Geometry check sheet. Reference: drawing and pictorial views, mm from the part's lowest x, y, z. Round coordinates to 2 decimals unless told otherwise and drop trailing zeros. Order: outer loops, then holes, each group sorted by start corner. A loop starts at its lowest first (then second) coordinate and runs counter-clockwise, first axis right, second up.
(1) Go/stop test with flat-tipped pins: pin 1 (5 mm diameter, centred on y = 16.5, z = 19, fed in from +X); pin 2 (2 mm diameter, centred on x = 36, z = 9, fed in from +Y); pin 3 (3 mm diameter, centred on x = 38.5, z = 3.5, fed in from -Y). Record where each tip stops, or that it passes through.
(2) Sectioned sample at A-A (x = 13). Record the boundary of the cut face in (y, z).
(3) Material ranges on line 1 along X through (y, z) = (9.25, 1.5) (1 decimal); line 2 along Z through (x, y) = (22, 12.5); line 3 along Z through (x, y) = (11.5, 13.5), recorded low to high.
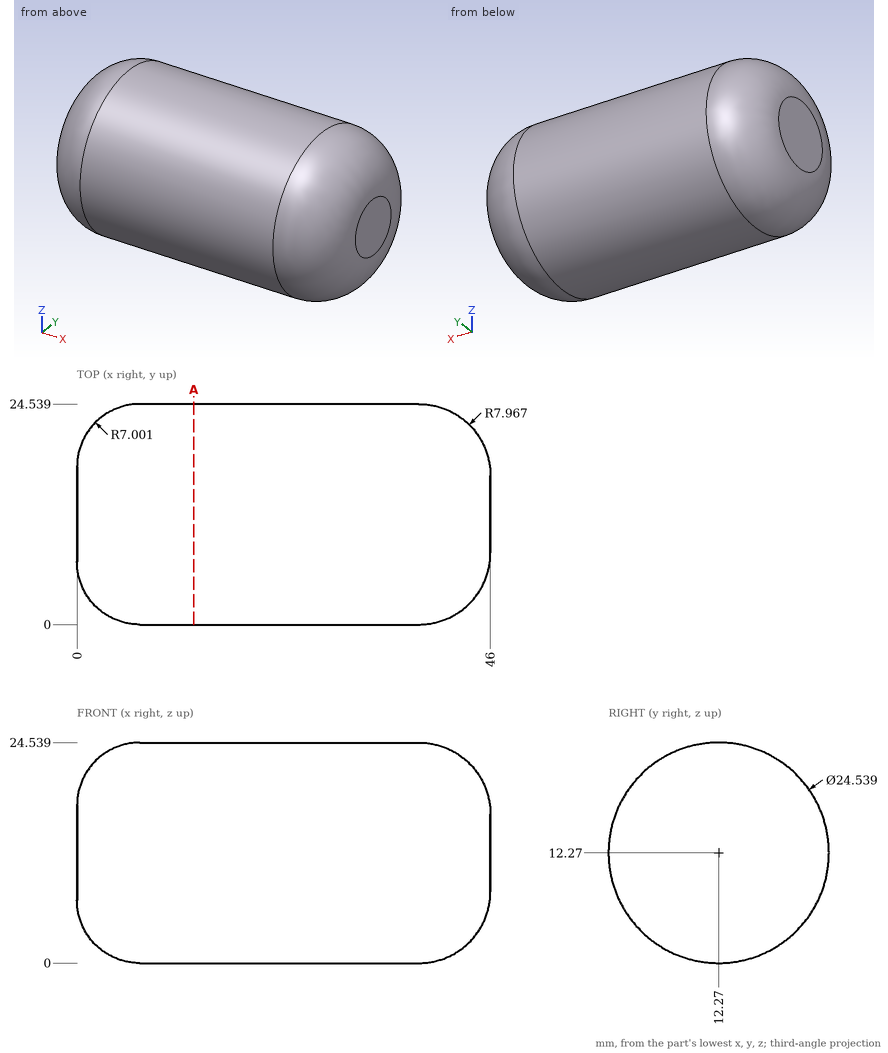
Answer below:
1. pin 1: stops at x = 45.92
1. pin 2: stops at y = 24.33
1. pin 3: stops at y = 2.4
2. outline: circle Ø24.54 at (12.27, 12.27)
3. line 1: x = 3.3 to 42
3. line 2: z = 0 to 24.54
3. line 3: z = 0.06 to 24.48
